```python
from build123d import *

# Parameters (mm, degrees)
SKETCH_1_W             = 50
SKETCH_1_H             = 1
SM_BASE_FLANGE_1_DEPTH = 160
OTHER_START            = -160
OTHER_1_DEPTH          = 320
OTHER_1_2_DEPTH        = 320
SKETCH_4_R             = 1.6
CUT_EXTRUDE_1_DEPTH    = 2


# Read off the part's stored shape, not the designer's step: 绘制的折弯1
# Sheet-metal steps are written as plain solids
with BuildPart() as part:
    # Sketch 1 → 基体-法兰1 (new, symmetric)
    with BuildSketch(Plane(origin=(0, 0, 0), x_dir=(0, 0, -1), z_dir=(1, 0, 0))):
        with Locations((-7, 22.5)):
            Rectangle(SKETCH_1_W, SKETCH_1_H)
    extrude(amount=SM_BASE_FLANGE_1_DEPTH, both=True)

    # Other 1 outline → Other 1 (cut)
    with BuildSketch(Plane.YZ.offset(OTHER_START)):
        with BuildLine():
            ThreePointArc((22, 15.2634), (22.271171885, 16.195226164), (23, 16.83604109))
            Line((23, 16.83604109), (23, 32))
            Line((23, 32), (22, 32))
            Line((22, 32), (22, 15.2634))
        make_face()
    extrude(amount=OTHER_1_DEPTH, mode=Mode.SUBTRACT)

    # Other 1 2 outline → Other 1 2 (add)
    with BuildSketch(Plane.YZ.offset(OTHER_START)):
        with BuildLine():
            ThreePointArc((23, 15.2634), (23.215745145, 15.784254855), (23.7366, 16))
            Line((23.7366, 16), (38.530753262, 16))
            Line((38.530753262, 16), (38.530753262, 17))
            Line((38.530753262, 17), (23.7366, 17))
            ThreePointArc((23.7366, 17), (23.359286442, 16.958514757), (23, 16.83604109))
            Line((23, 16.83604109), (23, 15.2634))
        make_face()
    extrude(amount=OTHER_1_2_DEPTH)

    # 草图4 → 切除-拉伸1 (cut)
    with BuildSketch(Plane(origin=(0, 0, 16), x_dir=(-1, 0, 0), z_dir=(0, 0, -1))):
        with Locations(Location((0, 31.530753262, 0), (0, 0, 90))):
            Circle(SKETCH_4_R)
        with Locations(Location((145, 31.530753262, 0), (0, 0, 90))):
            Circle(SKETCH_4_R)
        with Locations(Location((65, 31.530753262, 0), (0, 0, 90))):
            Circle(SKETCH_4_R)
        with Locations(Location((-145, 31.530753262, 0), (0, 0, 90))):
            Circle(SKETCH_4_R)
        with Locations(Location((-65, 31.530753262, 0), (0, 0, 90))):
            Circle(SKETCH_4_R)
    extrude(amount=-CUT_EXTRUDE_1_DEPTH, mode=Mode.SUBTRACT)


solid = part.part
```
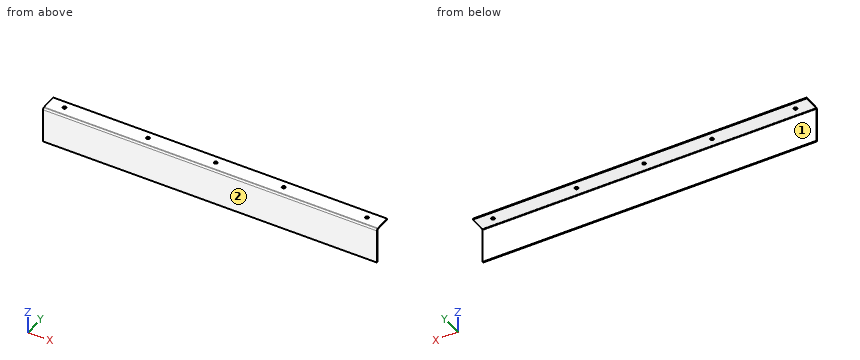
The model under review builds one solid part; all positions refer to its coordinate system, in mm. Face numbers are marked on the shaded views. A direction names the side the tool comes from. Round coordinates to 2 decimals unless told otherwise and drop trailing zeros. Loops run counter-clockwise (first coordinate to the right, second up) from the corner with the lowest first, then second, coordinate; pieces in that order, holes last.
Item 1: For line 1 (Y direction, x = -91, z = 14.5); line 2 (Z direction, x = -29, y = 24); line 3 (Y direction, x = 145, z = 16.4), list the stretches that pass through material, from the lowest coordinate up.
Determined:
line 1: y = 22 to 23
line 2: z = 16 to 17
line 3: y = 22.42 to 29.93, 33.13 to 38.53
Item 2: Take a section at B-B (z = -12.5). Write out the cut boundary in (x, y), then the cut area to 3 significant figures.
Determined:
outline: (-160, 22) - (160, 22) - (160, 23) - (-160, 23) - close
area: 320 mm2
Item 3: For the marked faces 1 and 2, list the 3-axis set-ups (+Z, -Z, +X, -X, +Y, -Y) from which the entire face can be reached by the end or side of a thin tool; tool diameter is ignored.
Determined:
face 1: -Z, +X, -X, +Y
face 2: +Z, -Z, +X, -X, -Y
Item 4: Take a section at A-A (x = -134). Write out the cut boundary in (y, z).
Determined:
outline: (22, -18) - (23, -18) - (23, 15.26) arc R0.74 cw to (23.74, 16) - (38.53, 16) - (38.53, 17) - (23.74, 17) arc R1.74 ccw to (22, 15.26) - close
Item 5: Clearance check with flat-ended pins moving along their axes: pin 1 Ø8 at (x, z) = (7.5, -0.5) entering from +Y; pin 2 Ø5 at (x, y) = (65, 31.53) entering from -Z. State where each tip first meets the part, or that it passes through.
Determined:
pin 1: stops at y = 23
pin 2: stops at z = 16
